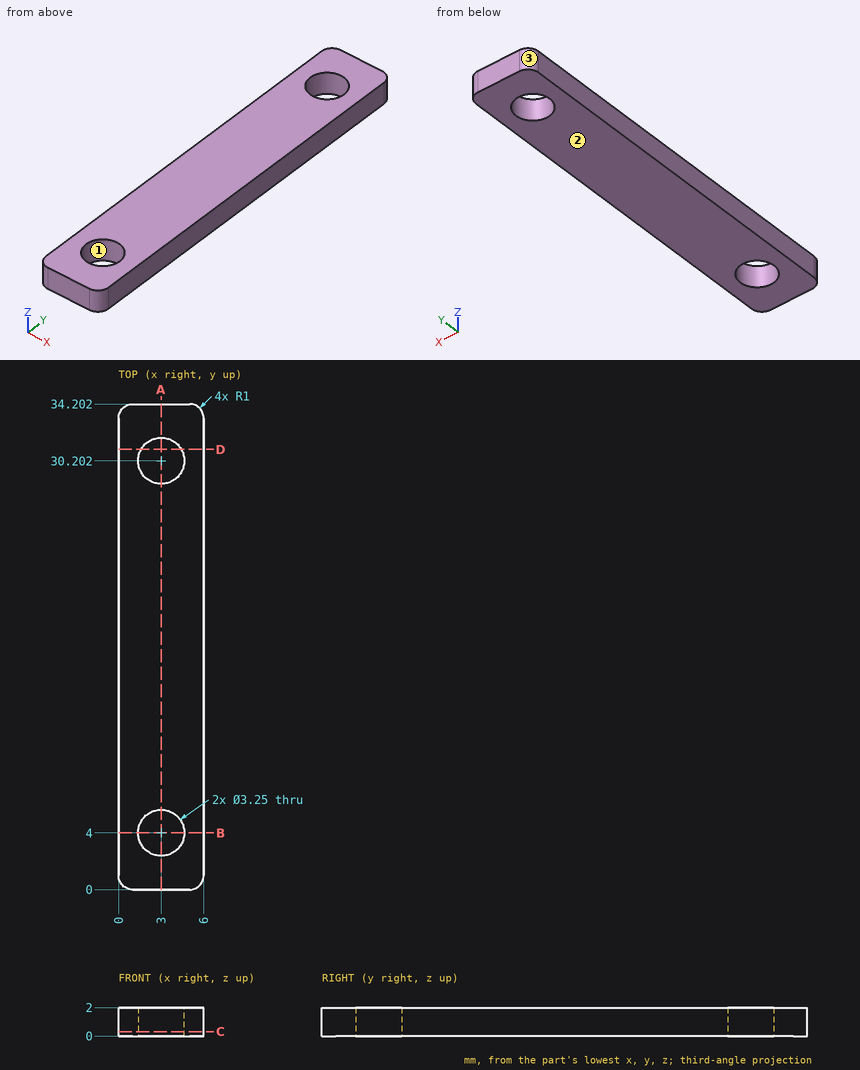
Input: dimensioned drawing with shaded views. Units: mm. Origin: part minimum x, y, z. Give positions to 0.01 mm unless a question says otherwise; leave off trailing zeros. Order: outer loops, then holes, each group sorted by start corner. A loop starts at its lowest first (then second) coordinate and runs counter-clockwise, first axis right, second up.
(1) Material intervals for line 1 along Y through (x, z) = (3, 0.6) (3 decimals); line 2 along X through (y, z) = (4, 1.1) (3 decimals); line 3 along X through (y, z) = (31.5, 0.1), sorted ascending.
(2) Contact query for a flat-ended pin moving along its axis: P1, Ø1.9, axis at x = 3, y = 4, coming from the -Z side. Output: stop coordinate, or through.
(3) Section query D-D (y = 31). Return the cut outline in (x, z).
(4) Section query C-C (z = 0.3). Return the cut outline in (x, y) (3 decimals).
(5) Pull-direction query (X, two-part tool) for the marked faces 1, 2 and 3; classes: +X half, -X half, draft (parallel to the pull), parting line (faces both ways), or undercut.
(6) Section query A-A (x = 3). Return the cut outline in (y, z) (3 decimals).
(7) Section query B-B (y = 4). Return the cut outline in (x, z) (3 decimals), plus the area to 3 significant figures.
Outcome:
1. line 1: y = 0 to 2.375, 5.625 to 28.577, 31.827 to 34.202
1. line 2: x = 0 to 1.375, 4.625 to 6
1. line 3: x = 0 to 2.02, 3.98 to 6
2. P1: passes through
3. outline: (0, 0) - (1.58, 0) - (1.58, 2) - (0, 2) - close; (4.42, 0) - (6, 0) - (6, 2) - (4.42, 2) - close
4. outline: (0, 1) arc R1 ccw to (1, 0) - (5, 0) arc R1 ccw to (6, 1) - (6, 33.202) arc R1 ccw to (5, 34.202) - (1, 34.202) arc R1 ccw to (0, 33.202) - close; hole circle Ø3.25 at (3, 4); hole circle Ø3.25 at (3, 30.202)
5. face 1: undercut
5. face 2: draft
5. face 3: -X half
6. outline: (0, 0) - (2.375, 0) - (2.375, 2) - (0, 2) - close; (5.625, 0) - (28.577, 0) - (28.577, 2) - (5.625, 2) - close; (31.827, 0) - (34.202, 0) - (34.202, 2) - (31.827, 2) - close
7. outline: (0, 0) - (1.375, 0) - (1.375, 2) - (0, 2) - close; (4.625, 0) - (6, 0) - (6, 2) - (4.625, 2) - close
7. area: 5.50 mm2
